The drawing under review shows one solid part. Ordinate dimensions are in mm from its lowest x, y, z. A direction names the side the tool comes from. Round coordinates to 2 decimals unless told otherwise and drop trailing zeros. Write each loop counter-clockwise with the first axis right and the second up, starting at its lowest first coordinate (ties: lowest second). Pieces come first, ordered by that corner, then holes. Notation, with made-up numbers: (69.5, -24.75) -> (100.5, -24.75) arc R20 cw to (100.5, 10.25) -> close; hole circle Ø6 at (-20.5, 8). An arc over 180 degrees is marked (long way). Write item = value, one per line. Start each with the question number.
Item 1: To check wall thickness, follow L1, parallel to Z at x = 3.75, y = 1.75 (1 decimal); L2, parallel to Z at x = 3.25, y = 1.75 (1 decimal); L3, parallel to Y at x = 0.75, z = 7.75. State the ranges of each line that lie inside material, in increasing order.
Item 2: Add section D-D, the plane z = 7. State the section outline as (x, y) points, then the cut area to 3 significant figures.
Item 3: For pin 1 Ø3 at (x, z) = (4.5, 14.5) entering from +Y; pin 2 Ø2.5 at (x, z) = (3.05, 12.21) entering from +Y; pin 3 Ø3 at (x, y) = (1.5, 7) entering from +Z, all flat-tipped, find the tip position at first contact; note any pin that passes through.
Item 4: Add section B-B, the plane y = 2.5. State how many separate pieces and enclosed holes the cut face has, then the cut area to 3 significant figures.
Item 5: Machinability: for the marked faces 4 and 5, which of the approach directions +Z, -Z, +X, -X, +Y, -Y give a long, thin tool a straight path to every point of the face, cutting with its end or side? Answer none if there is none.
Item 6: Mouldability with a two-part tool opening along X and no side actions: class the marked faces 1, 2 and 3 as released by +X, released by -X, zero draft, split by the parting line, or undercut.
Item 7: Add section C-C, the plane y = 13.75. State the section outline as (x, z) points.
Item 8: Add section A-A, the plane x = 1. State the section outline as (y, z) points.
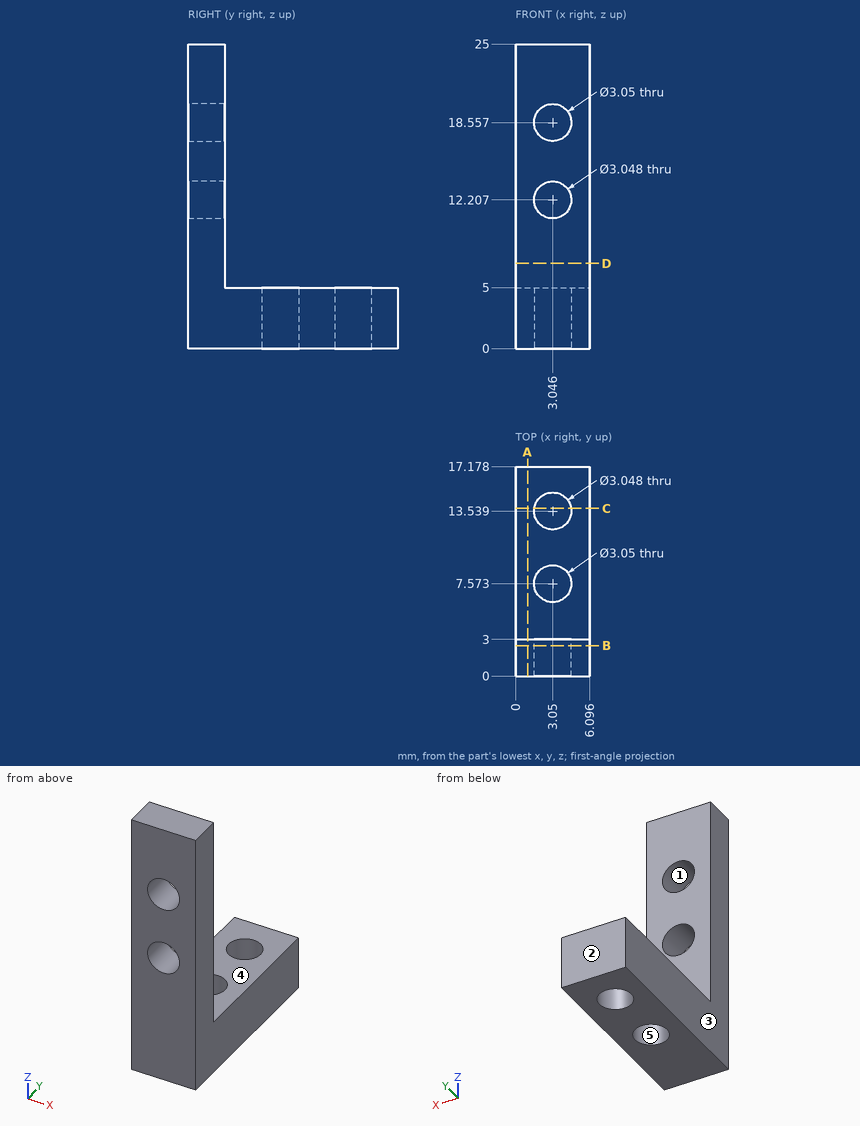
Result set:
q1.L1 = 0 to 10.9, 13.6 to 17.2, 19.9 to 25
q1.L2 = 0 to 10.7, 13.7 to 17, 20.1 to 25
q1.L3 = 0 to 3
q2.outline = (0, 0) -> (6.1, 0) -> (6.1, 3) -> (0, 3) -> close
q2.area = 18.3 mm²
q3.pin_1 = 3
q3.pin_2 = through
q3.pin_3 = 5
q4.separate_pieces = 1
q4.enclosed_holes = 2
q4.area = 138 mm²
q5.face_4 = +Z, +X, -X, +Y
q5.face_5 = +Z, -Z
q6.face_1 = undercut
q6.face_2 = zero draft
q6.face_3 = released by -X
q7.outline = (0, 0) -> (1.54, 0) -> (1.54, 5) -> (0, 5) -> close; (4.56, 0) -> (6.1, 0) -> (6.1, 5) -> (4.56, 5) -> close
q8.outline = (0, 0) -> (17.18, 0) -> (17.18, 5) -> (3, 5) -> (3, 25) -> (0, 25) -> close
